Can you work these out from the model? Positions are in its coordinate system, mm. A direction names the side the tool comes from. Round coordinates to 2 decimals unless told otherwise and drop trailing zeros. Write each loop counter-clockwise with the first axis right and the second up, starting at its lowest first coordinate (ties: lowest second). Pieces come first, ordered by that corner, then holes.
Q1. If we section it at C-C (x = 25.4): Please give me the cut outline in (y, z) (1 decimal), plus the area to 3 significant figures.
Q2. If we section it at A-A (y = 304.8): Please give me the cut outline in (x, z) (1 decimal).
Q3. We'd pull the mould along Y, two halves only. Please class faces 1 (the cylindrical face through (22.303, 290.852, -23.79)), 2 (the flat face through (25, 330.2, -23)), 3 (the flat face through (25, 163, 0)): +Y half, -Y half, draft (parallel to the pull), parting line (faces both ways), or undercut.
Q4. If we section it at B-B (z = -19.25): Please give me the cut outline in (x, y) (3 decimals), plus the area to 3 significant figures.
Q5. I'm going to push a flat-ended pin straight in: pin 1 Ø5 at (y, z) = (19.05, -12.7) entering from +X (3 decimals). Where does the tip first touch, or does it pass through?
Q6. If we section it at D-D (y = 59): Please give me the cut outline in (x, z) (3 decimals), plus the area to 3 significant figures.
Q7. Please list where these lines run through material, in increasing order: line 1 along Y through (x, z) = (48.55, -12.7); line 2 along Z through (x, y) = (24.5, 73) (3 decimals); line 3 along X through (y, z) = (128.5, -18) (3 decimals).
Q8. For faces 4 (the flat face through (0, 163, -13)), 5 (the cylindrical face through (49.235, 18.029, -15.164)), 6 (the flat face through (3.175, 163, -13)), which set-ups out of +Z, -Z, +X, -X, +Y, -Y let a thin tool reach every point of the face, with its end or its side?
from build123d import *

# Parameters (mm, degrees)
SKETCH1_W           = 50.8
SKETCH1_H           = 25.4
SKETCH1_W_2         = 44.45
SKETCH1_H_2         = 19.05
BOSS_EXTRUDE2_DEPTH = 330.2
SKETCH2_R           = 14.2875
CUT_EXTRUDE1_DEPTH  = 25.4
SKETCH3_R           = 2.667
CUT_EXTRUDE2_DEPTH  = 3.175


with BuildPart() as part:
    # Sketch1 → Boss-Extrude2 (new body)
    with BuildSketch(Plane(origin=(0, 0, 0), x_dir=(1, 0, 0), z_dir=(0, 1, 0))):
        with Locations((25.4, 12.7)):
            Rectangle(SKETCH1_W, SKETCH1_H)
        with Locations((25.4, 12.7)):
            Rectangle(SKETCH1_W_2, SKETCH1_H_2, mode=Mode.SUBTRACT)
    extrude(amount=BOSS_EXTRUDE2_DEPTH)

    # Sketch2 → Cut-Extrude1 (cut)
    with BuildSketch(Plane.XY):
        with Locations((25.4, 304.8)):
            Circle(SKETCH2_R)
    extrude(amount=-CUT_EXTRUDE1_DEPTH, mode=Mode.SUBTRACT)

    # Sketch3 → Cut-Extrude2 (cut)
    with BuildSketch(Plane(origin=(50.8, 0, 0), x_dir=(0, 0, -1), z_dir=(1, 0, 0))):
        with Locations((12.7, 19.05)):
            Circle(SKETCH3_R)
        with Locations((12.7, 6.35)):
            Circle(SKETCH3_R)
    extrude(amount=-CUT_EXTRUDE2_DEPTH, mode=Mode.SUBTRACT)


solid = part.part
A:
1. outline: (0, -25.4) - (290.5, -25.4) - (290.5, -22.2) - (0, -22.2) - close; (0, -3.2) - (290.5, -3.2) - (290.5, 0) - (0, 0) - close; (319.1, -25.4) - (330.2, -25.4) - (330.2, -22.2) - (319.1, -22.2) - close; (319.1, -3.2) - (330.2, -3.2) - (330.2, 0) - (319.1, 0) - close
1. area: 1,920 mm2
2. outline: (0, -25.4) - (11.1, -25.4) - (11.1, -22.2) - (3.2, -22.2) - (3.2, -3.2) - (11.1, -3.2) - (11.1, 0) - (0, 0) - close; (39.7, -25.4) - (50.8, -25.4) - (50.8, 0) - (39.7, 0) - (39.7, -3.2) - (47.6, -3.2) - (47.6, -22.2) - (39.7, -22.2) - close
3. face 1: undercut
3. face 2: +Y half
3. face 3: draft
4. outline: (0, 0) - (3.175, 0) - (3.175, 330.2) - (0, 330.2) - close; (47.625, 0) - (50.8, 0) - (50.8, 330.2) - (47.625, 330.2) - close
4. area: 2,100 mm2
5. pin 1: stops at x = 3.175
6. outline: (0, -25.4) - (50.8, -25.4) - (50.8, 0) - (0, 0) - close; hole (3.175, -22.225) - (47.625, -22.225) - (47.625, -3.175) - (3.175, -3.175) - close
6. area: 444 mm2
7. line 1: y = 0 to 3.68, 9.02 to 16.38, 21.72 to 330.2
7. line 2: z = -25.4 to -22.225, -3.175 to 0
7. line 3: x = 0 to 3.175, 47.625 to 50.8
8. face 4: +Z, -Z, -X, +Y, -Y
8. face 5: +X
8. face 6: +Y, -Y
